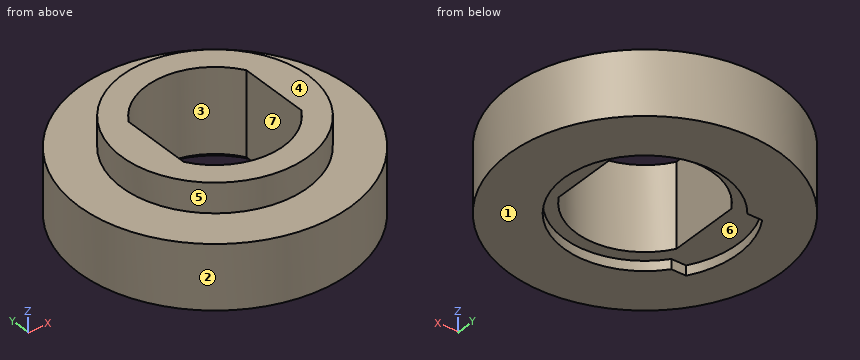
from build123d import *

# Parameters (mm, degrees)
F3_DEPTH = 25
F5_DEPTH = 2


with BuildPart() as f1:
    # F0 (on Front) → F1 (revolve)
    with BuildSketch(Plane.XZ):
        Polygon((19, 0), (0, 0), (0, -17), (16.5, -17), (16.5, -19), (27.75, -19), (27.75, -6), (19, -6), align=None)
    revolve(axis=Axis((0, 0, 0.8052456426), (0, 0, -1)))

    # F2 (on face) → F3 (cut)
    with BuildSketch(Plane.XY):
        with BuildLine():
            Line((-12, 7.2111025509), (-12, -7.2111025509))
            ThreePointArc((-12, -7.2111025509), (0, -14), (12, -7.2111025509))
            Line((12, -7.2111025509), (12, 7.2111025509))
            ThreePointArc((12, 7.2111025509), (0, 14), (-12, 7.2111025509))
        make_face()
    extrude(amount=-F3_DEPTH, mode=Mode.SUBTRACT)

    # F4 (on face) → F5 (cut, through all)
    with BuildSketch(Plane(origin=(0, 0, -19), x_dir=(1, 0, 0), z_dir=(0, 0, -1))):
        with BuildLine():
            Line((-13.1244047484, 10), (-16.1554944214, 10))
            ThreePointArc((-16.1554944214, 10), (-19, 0), (-16.1554944214, -10))
            Line((-16.1554944214, -10), (-13.1244047484, -10))
            ThreePointArc((-13.1244047484, -10), (-16.5, 0), (-13.1244047484, 10))
        make_face()
    extrude(amount=-F5_DEPTH, mode=Mode.SUBTRACT)


solid = f1.part
Design review of the part built by this model. Coordinates are the model's own, in mm. Face numbers are marked on the shaded views. A direction names the side the tool comes from. Give positions to 0.01 mm unless a question says otherwise; leave off trailing zeros. Write each loop counter-clockwise with the first axis right and the second up, starting at its lowest first coordinate (ties: lowest second). Pieces come first, ordered by that corner, then holes. Notation, with made-up numbers: M 71.5,49 L 85.5,49 A17 cw 85.5,56 Z; hole C 69,5.5 d2. An arc over 180 degrees is marked long. Return JSON: item names as keys, results as strings. Group by question number.
Item 1: The part is to be moulded in two halves that separate along Y. For the marked faces 1, 2 and 3, say which applies: pulls with the +Y half, pulls with the -Y half, needs draft (parallel to the pull), parting line crosses it, or undercut.
Item 2: Take a section at C-C (x = 6). Give the boundary of the cut face in (y, z), plus the area to 3 significant figures.
Item 3: Take a section at D-D (z = -17.75). Give the boundary of the cut face in (x, y).
Item 4: Take a section at A-A (y = 0). Give the boundary of the cut face in (x, z), plus the area to 4 significant figures.
Item 5: Take a section at B-B (z = -13.5). Give the boundary of the cut face in (x, y), plus the area to 3 significant figures.
Item 6: Tool access review of the marked faces 4, 5, 6 and 7: name each direction out of +Z, -Z, +X, -X, +Y, -Y from which nothing blocks a thin tool from reaching the whole face with its end or side.
Item 7: Wall thickness on line 1 along Y through (x, z) = (0, -18.3); line 2 along Y through (x, z) = (0.5, -14); line 3 along Z through (x, y) = (18.5, 15.5): over which ranges is each line inside the solid? List them lowest first.
Item 8: Clearance check with flat-ended pins moving along their axes: pin 1 Ø2 at (y, z) = (-20.5, -13) entering from +X; pin 2 Ø1.5 at (x, z) = (-19, -14.5) entering from -Y; pin 3 Ø0.6 at (x, z) = (-15, -18) entering from +Y. State where each tip first meets the part, or that it passes through.
Return value:
{
 "1": {"face 1": "needs draft", "face 2": "parting line crosses it", "face 3": "undercut"},
 "2": {"outline": "M -27.09,-19 L -15.37,-19 L -15.37,-17 L -12.65,-17 L -12.65,0 L -18.03,0 L -18.03,-6 L -27.09,-6 Z; M 12.65,-17 L 15.37,-17 L 15.37,-19 L 27.09,-19 L 27.09,-6 L 18.03,-6 L 18.03,0 L 12.65,0 Z", "area": "429 mm2"},
 "3": {"outline": "C 0,0 d55.5; hole M -16.16,-10 L -13.12,-10 A16.5 ccw long -13.12,10 L -16.16,10 A19 ccw Z"},
 "4": {"outline": "M -27.75,-19 L -19,-19 L -19,-17 L -12,-17 L -12,0 L -19,0 L -19,-6 L -27.75,-6 Z; M 12,-17 L 16.5,-17 L 16.5,-19 L 27.75,-19 L 27.75,-6 L 19,-6 L 19,0 L 12,0 Z", "area": "470.5 mm2"},
 "5": {"outline": "C 0,0 d55.5; hole M -12,-7.21 A14 ccw 12,-7.21 L 12,7.21 A14 ccw -12,7.21 Z", "area": "1,840 mm2"},
 "6": {"face 4": "+Z, +X, -X, +Y, -Y", "face 5": "+Z", "face 6": "-Z", "face 7": "+Z, -Z"},
 "7": {"line 1": "y = -27.75 to -16.5, 16.5 to 27.75", "line 2": "y = -27.75 to -13.99, 13.99 to 27.75", "line 3": "z = -19 to -6"},
 "8": {"pin 1": "stops at x = 19.74", "pin 2": "stops at y = -20.9", "pin 3": "stops at y = 23.54"}
}
